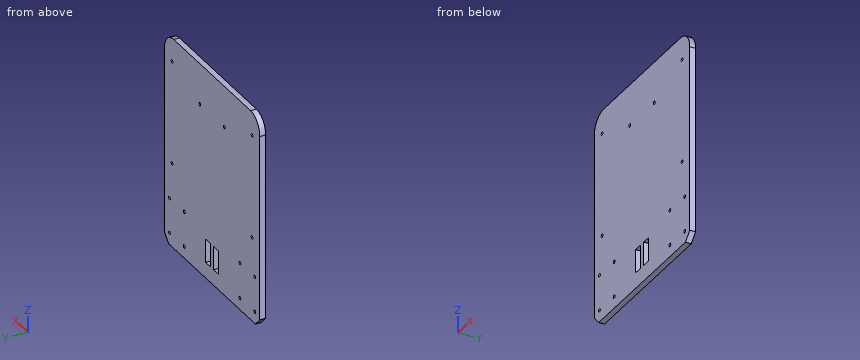
```python
from build123d import *

# Parameters (mm, degrees)
SKETCH7_W           = 155
SKETCH7_H           = 180
BOSS_EXTRUDE2_DEPTH = 5
SKETCH8_R           = 1.4
CUT_EXTRUDE3_DEPTH  = 5
SKETCH9_R           = 1.4
CUT_EXTRUDE4_DEPTH  = 5
CUT_EXTRUDE5_DEPTH  = 5
SKETCH11_W          = 8
SKETCH11_H          = 20
CUT_EXTRUDE6_DEPTH  = 5
CUT_EXTRUDE7_DEPTH  = 5
SKETCH15_R          = 1.4
CUT_EXTRUDE8_DEPTH  = 10


with BuildPart() as part:
    # Sketch7 → Boss-Extrude2 (new body)
    with BuildSketch(Plane(origin=(0, 0, 0), x_dir=(1, 0, 0), z_dir=(0, 1, 0))):
        Rectangle(SKETCH7_W, SKETCH7_H)
    extrude(amount=BOSS_EXTRUDE2_DEPTH)

    # Sketch8 → Cut-Extrude3 (cut)
    with BuildSketch(Plane(origin=(0, 5, 0), x_dir=(1, 0, 0), z_dir=(0, 1, 0))):
        with Locations(Location((-69.25, 80, 0), (0, 0, 270))):
            Circle(SKETCH8_R)
        with Locations(Location((-69.25, 50, 0), (0, 0, 270))):
            Circle(SKETCH8_R)
        with Locations(Location((-45.25, 50, 0), (0, 0, 270))):
            Circle(SKETCH8_R)
        with Locations(Location((-45.25, 80, 0), (0, 0, 270))):
            Circle(SKETCH8_R)
        with Locations(Location((45.25, 80, 0), (0, 0, 90))):
            Circle(SKETCH8_R)
        with Locations(Location((45.25, 50, 0), (0, 0, 90))):
            Circle(SKETCH8_R)
        with Locations(Location((69.25, 50, 0), (0, 0, 90))):
            Circle(SKETCH8_R)
        with Locations(Location((69.25, 80, 0), (0, 0, 90))):
            Circle(SKETCH8_R)
    extrude(amount=-CUT_EXTRUDE3_DEPTH, mode=Mode.SUBTRACT)

    # Sketch9 → Cut-Extrude4 (cut)
    with BuildSketch(Plane(origin=(0, 5, 0), x_dir=(1, 0, 0), z_dir=(0, 1, 0))):
        with Locations(Location((-65, 18, 0), (0, 0, 270))):
            Circle(SKETCH9_R)
        with Locations(Location((65, 18, 0), (0, 0, 90))):
            Circle(SKETCH9_R)
        with Locations(Location((-65, -70, 0), (0, 0, 270))):
            Circle(SKETCH9_R)
        with Locations(Location((65, -70, 0), (0, 0, 90))):
            Circle(SKETCH9_R)
    extrude(amount=-CUT_EXTRUDE4_DEPTH, mode=Mode.SUBTRACT)

    # Sketch10 → Cut-Extrude5 (cut)
    with BuildSketch(Plane(origin=(0, 5, 0), x_dir=(1, 0, 0), z_dir=(0, 1, 0))):
        with BuildLine():
            Line((-77.5, -90), (-62.5, -90))
            ThreePointArc((-62.5, -90), (-73.106601718, -85.606601718), (-77.5, -75))
            Line((-77.5, -75), (-77.5, -90))
        make_face()
        with BuildLine():
            Line((77.5, -90), (77.5, -75))
            ThreePointArc((77.5, -75), (73.106601718, -85.606601718), (62.5, -90))
            Line((62.5, -90), (77.5, -90))
        make_face()
    extrude(amount=-CUT_EXTRUDE5_DEPTH, mode=Mode.SUBTRACT)

    # Sketch11 → Cut-Extrude6 (cut)
    with BuildSketch(Plane(origin=(0, 5, 0), x_dir=(1, 0, 0), z_dir=(0, 1, 0))):
        with Locations((6.5, 66.58550083)):
            Rectangle(SKETCH11_W, SKETCH11_H)
        with Locations((-6.5, 66.58550083)):
            Rectangle(SKETCH11_W, SKETCH11_H)
    extrude(amount=-CUT_EXTRUDE6_DEPTH, mode=Mode.SUBTRACT)

    # Sketch13 → Cut-Extrude7 (cut)
    with BuildSketch(Plane(origin=(0, 5, 0), x_dir=(1, 0, 0), z_dir=(0, 1, 0))):
        Polygon((-70.5, 90), (-77.5, 83), (-77.5, 90), align=None)
        Polygon((70.5, 90), (77.5, 83), (77.5, 90), align=None)
    extrude(amount=-CUT_EXTRUDE7_DEPTH, mode=Mode.SUBTRACT)

    # Sketch15 → Cut-Extrude8 (cut)
    with BuildSketch(Plane(origin=(0, 5, 0), x_dir=(1, 0, 0), z_dir=(0, 1, 0))):
        with Locations(Location((-20, -55, 0), (0, 0, 270))):
            Circle(SKETCH15_R)
        with Locations(Location((20, -55, 0), (0, 0, 270))):
            Circle(SKETCH15_R)
    extrude(amount=-CUT_EXTRUDE8_DEPTH, mode=Mode.SUBTRACT)


solid = part.part
```
Could you check a few things on this model? Use its own coordinates, in mm. Give positions to 0.01 mm unless a question says otherwise; leave off trailing zeros. Loops run counter-clockwise (first coordinate to the right, second up) from the corner with the lowest first, then second, coordinate; pieces in that order, holes last. Notation, with made-up numbers: (25, 45.5) - (38, 45.5) arc R19 ccw to (38, 66.5) - close; hole circle Ø9 at (-26, 10.5). An arc over 180 degrees is marked (long way). Answer in a Markdown table with one row per item. Add a question column.
Q1. Please list where these lines run through material, in increasing order: L1, parallel to Z at x = 45.25, y = 3.3; L2, parallel to X at y = 2.8, z = -80; L3, parallel to X at y = 2.9, z = -18. Write a range as from..to.
Q2. If we section it at B-B (y = 1.9): State how many separate pieces and enclosed holes the cut face has, plus the area to 3 significant figures.
Q3. For pin 1 (3.5 mm diameter, centred on x = 45.25, z = -50, fed in from +Y), with a flat end and sliding along its axis, tell me the tip position at first contact or that it passes through.
Q4. If we section it at A-A (z = -69.5): List the corners of the cut face in (x, y) for me.
The answers:
| question | item | result |
|---|---|---|
| 1 | L1 | z = -90..-81.4, -78.6..-51.4, -48.6..90 |
| 1 | L2 | x = -77.5..-70.65, -67.85..-46.65, -43.85..43.85, 46.65..67.85, 70.65..77.5 |
| 1 | L3 | x = -77.5..-66.4, -63.6..63.6, 66.4..77.5 |
| 2 | separate pieces | 1 |
| 2 | enclosed holes | 16 |
| 2 | area | 27,300 mm^2 |
| 3 | pin 1 | stops at y = 5 |
| 4 | outline | (-77.5, 0) - (-10.5, 0) - (-10.5, 5) - (-77.5, 5) - close; (-2.5, 0) - (2.5, 0) - (2.5, 5) - (-2.5, 5) - close; (10.5, 0) - (77.5, 0) - (77.5, 5) - (10.5, 5) - close |
